The model under review builds one solid part; all positions refer to its coordinate system, in mm. Face numbers are marked on the shaded views. A direction names the side the tool comes from. Coordinates: 2 decimals unless noted, no trailing zeros. Order: outer loops, then holes, each group sorted by start corner. A loop starts at its lowest first (then second) coordinate and runs counter-clockwise, first axis right, second up. Notation, with made-up numbers: M 5,65.5 L 34,65.5 A10 ccw 34,83.5 Z; hole C -6.75,7 d1. An arc over 180 degrees is marked long. One line per item, written item: value.
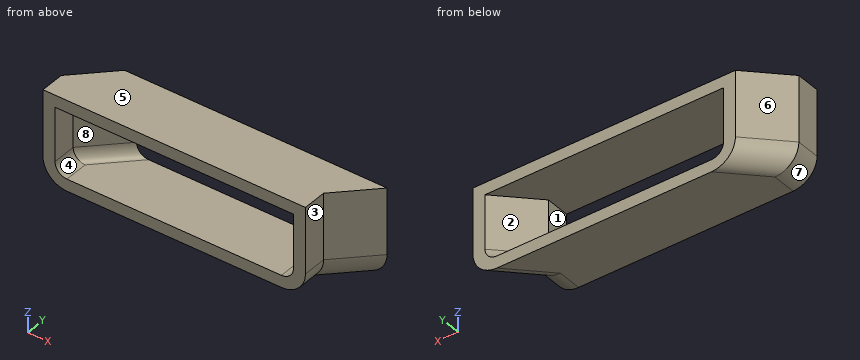
```python
from build123d import *

# Parameters (mm, degrees)
EXTRUDE_2_DEPTH = 2


with BuildPart() as part:
    # По траектории1: sweep along a path in Эскиз2
    with BuildLine(Plane.XY) as sweep_1_path:
        Line((-13.420763014, 0), (-10.40702754, 3.013735474))
    # Эскиз1 → По траектории1 (sweep)
    with BuildSketch(Plane(origin=(0, 0, 0), x_dir=(1, 0, 0), z_dir=(0, 1, 0))):
        with BuildLine():
            Line((-11.420763014, 2.209655172), (6.479236986, 2.209655172))
            ThreePointArc((6.479236986, 2.209655172), (7.893450549, 1.623868735), (8.479236986, 0.209655172))
            Line((8.479236986, 0.209655172), (8.479236986, -5.290344828))
            Line((8.479236986, -5.290344828), (-13.420763014, -5.290344828))
            Line((-13.420763014, -5.290344828), (-13.420763014, 0.209655172))
            ThreePointArc((-13.420763014, 0.209655172), (-12.834976576, 1.623868735), (-11.420763014, 2.209655172))
        make_face()
        with BuildLine():
            Line((-11.420763014, 1.209655172), (6.479236986, 1.209655172))
            ThreePointArc((6.479236986, 1.209655172), (7.186343768, 0.916761954), (7.479236986, 0.209655172))
            Line((7.479236986, 0.209655172), (7.479236986, -4.290344828))
            Line((7.479236986, -4.290344828), (-12.420763014, -4.290344828))
            Line((-12.420763014, -4.290344828), (-12.420763014, 0.209655172))
            ThreePointArc((-12.420763014, 0.209655172), (-12.127869795, 0.916761954), (-11.420763014, 1.209655172))
        make_face(mode=Mode.SUBTRACT)
    sweep(path=sweep_1_path.line)

    # Эскиз3 → Бобышка-Вытянуть2 (add)
    with BuildSketch(Plane.XZ):
        with BuildLine():
            Line((8.479236986, -0.209655172), (8.479236986, 5.290344828))
            Line((8.479236986, 5.290344828), (-13.420763014, 5.290344828))
            Line((-13.420763014, 5.290344828), (-13.420763014, -0.209655172))
            ThreePointArc((-13.420763014, -0.209655172), (-12.834976576, -1.623868735), (-11.420763014, -2.209655172))
            Line((-11.420763014, -2.209655172), (6.479236986, -2.209655172))
            ThreePointArc((6.479236986, -2.209655172), (7.893450549, -1.623868735), (8.479236986, -0.209655172))
        make_face()
        with BuildLine():
            Line((7.479236986, -0.209655172), (7.479236986, 4.290344828))
            Line((7.479236986, 4.290344828), (-12.420763014, 4.290344828))
            Line((-12.420763014, 4.290344828), (-12.420763014, -0.209655172))
            ThreePointArc((-12.420763014, -0.209655172), (-12.127869795, -0.916761954), (-11.420763014, -1.209655172))
            Line((-11.420763014, -1.209655172), (6.479236986, -1.209655172))
            ThreePointArc((6.479236986, -1.209655172), (7.186343768, -0.916761954), (7.479236986, -0.209655172))
        make_face(mode=Mode.SUBTRACT)
    extrude(amount=EXTRUDE_2_DEPTH)


solid = part.part
```
(1) Insertion check: pin 1 Ø1.6 at (y, z) = (-1.5, 1) entering from +X. The pin has a flat end and moves straight along its axis. Give the tip position at first contact, or say it passes through.
Geometry results:
pin 1: stops at x = 8.48
(2) Mouldability with a two-part tool opening along Z and no side actions: class the marked faces 5, 6, 7 and 8 as +Z half, -Z half, draft (parallel to the pull), parting line (faces both ways), or undercut.
Geometry results:
face 5: +Z half
face 6: draft
face 7: -Z half
face 8: undercut
(3) We need section B-B, the plane x = -0.5. State the section outline as (y, z) points, plus the area to 3 significant figures.
Geometry results:
outline: M -2,-2.21 L 3.01,-2.21 L 3.01,-1.21 L -2,-1.21 Z; M -2,4.29 L 3.01,4.29 L 3.01,5.29 L -2,5.29 Z
area: 10.0 mm2
(4) We need section A-A, the plane z = 2.5. State the section outline as (x, y) points, plus the area to 3 significant figures.
Geometry results:
outline: M -13.42,-2 L -12.42,-2 L -12.42,0 L -9.41,3.01 L -10.41,3.01 L -13.42,0 Z; M 7.48,-2 L 8.48,-2 L 8.48,0 L 11.49,3.01 L 10.49,3.01 L 7.48,0 Z
area: 10.0 mm2
(5) Tool access review of the marked faces 1, 2, 3 and 4: name each direction out of +Z, -Z, +X, -X, +Y, -Y from which nothing blocks a thin tool from reaching the whole face with its end or side.
Geometry results:
face 1: +Y, -Y
face 2: +Y
face 3: +Z, -Z, +X, -Y
face 4: -Y
(6) For L1, parallel to Z at x = -3.75, y = 1.1; L2, parallel to X at y = -1.2, z = 0.5; L3, parallel to X at y = 1.5, z = 2.5, list the stretches that pass through material, from the lowest coordinate up.
Geometry results:
L1: z = -2.21 to -1.21, 4.29 to 5.29
L2: x = -13.42 to -12.42, 7.48 to 8.48
L3: x = -11.92 to -10.92, 8.98 to 9.98
(7) We need section C-C, the plane y = -0.6. State the section outline as (x, z) points, plus the area to 3 significant figures.
Geometry results:
outline: M -13.42,-0.21 A2 ccw -11.42,-2.21 L 6.48,-2.21 A2 ccw 8.48,-0.21 L 8.48,5.29 L -13.42,5.29 Z; hole M -12.42,-0.21 A1 ccw -11.42,-1.21 L 6.48,-1.21 A1 ccw 7.48,-0.21 L 7.48,4.29 L -12.42,4.29 Z
area: 53.5 mm2
